Geometry check sheet. Reference: drawing and pictorial views, mm from the part's lowest x, y, z. A direction names the side the tool comes from. Round coordinates to 2 decimals unless told otherwise and drop trailing zeros. Order: outer loops, then holes, each group sorted by start corner. A loop starts at its lowest first (then second) coordinate and runs counter-clockwise, first axis right, second up.
Q1. Depth check by flat-ended pin: P1, Ø4, axis at x = 23, z = 17.5, coming from the +Y side. Enter the tip coordinate at first touch or a pass-through.
Q2. Set-up check for the marked faces 4 and 5: record each of +Z, -Z, +X, -X, +Y, -Y from which the full face is reachable in a straight line by a thin tool's end or side.
Q3. Cross-section at D-D on z = 16.75. Record the cut outline in (x, y).
Q4. Scan lines: probe 1 along X at (y, z) = (38.5, 3.75); probe 2 along X at (y, z) = (1.2, 10); probe 3 along Y at (x, z) = (0.8, 10). Record each from-to range of solid material in increasing order.
Q5. Cross-section at B-B on y = 24. Record the cut outline in (x, z), then the cut area to 3 significant figures.
Q6. Cross-section at C-C on y = 30. Record the cut outline in (x, z), then the cut area to 3 significant figures.
Q7. Cross-section at A-A on x = 27.5. Record the cut outline in (y, z), then the cut area to 3 significant figures.
Q8. Mould release check, pull along X, two halves, no side actions. Record for the marked faces 1, 2 and 3: +X half, -X half, draft (parallel to the pull), parting line (faces both ways), or undercut.
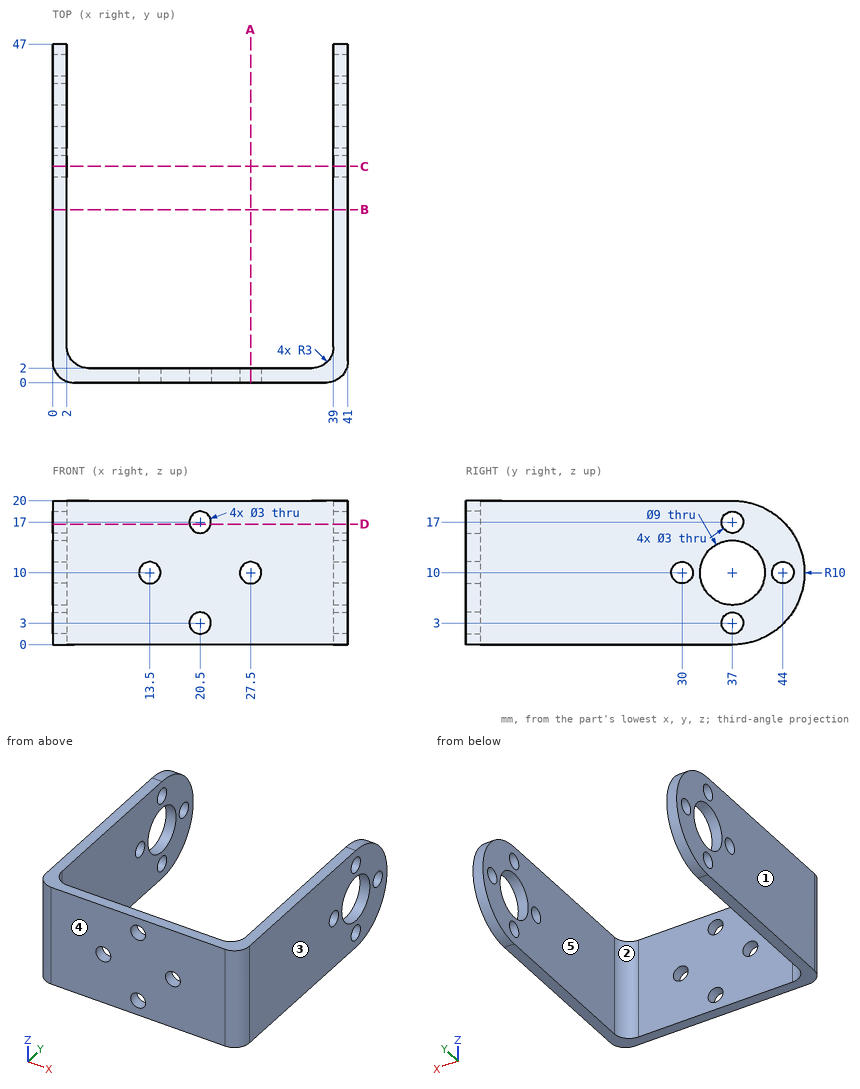
Results found:
1. P1: stops at y = 2
2. face 4: +Z, -Z, +X, -X, -Y
2. face 5: +Z, -Z, +Y
3. outline: (0, 3) arc R3 ccw to (3, 0) - (19.02, 0) - (19.02, 2) - (5, 2) arc R3 cw to (2, 5) - (2, 35.52) - (0, 35.52) - close; (0, 38.48) - (2, 38.48) - (2, 44.38) - (0, 44.38) - close; (21.98, 0) - (38, 0) arc R3 ccw to (41, 3) - (41, 35.52) - (39, 35.52) - (39, 5) arc R3 cw to (36, 2) - (21.98, 2) - close; (39, 38.48) - (41, 38.48) - (41, 44.38) - (39, 44.38) - close
4. probe 1: x = 0 to 2, 39 to 41
4. probe 2: x = 0.6 to 12, 15 to 26, 29 to 40.4
4. probe 3: y = 0.96 to 28.5, 31.5 to 32.5, 41.5 to 42.5, 45.5 to 47
5. outline: (0, 0) - (2, 0) - (2, 20) - (0, 20) - close; (39, 0) - (41, 0) - (41, 20) - (39, 20) - close
5. area: 80.0 mm2
6. outline: (0, 0) - (2, 0) - (2, 8.5) - (0, 8.5) - close; (0, 11.5) - (2, 11.5) - (2, 20) - (0, 20) - close; (39, 0) - (41, 0) - (41, 8.5) - (39, 8.5) - close; (39, 11.5) - (41, 11.5) - (41, 20) - (39, 20) - close
6. area: 68.0 mm2
7. outline: (0, 0) - (2, 0) - (2, 8.5) - (0, 8.5) - close; (0, 11.5) - (2, 11.5) - (2, 20) - (0, 20) - close
7. area: 34.0 mm2
8. face 1: -X half
8. face 2: undercut
8. face 3: +X half
